```python
from build123d import *

# Parameters (mm, degrees)
SKETCH1_W                = 30
SKETCH1_H                = 30
BOSS_EXTRUDE1_DEPTH      = 30
SKETCH2_R                = 3.375
CUT_EXTRUDE1_DEPTH       = 64.639610307
FILLET1_R                = 2.5
CUT_EXTRUDE2_DEPTH       = 64.639610307
CIRPATTERN1_COUNT        = 4
CIRPATTERN1_COPY_1_DEPTH = 64.639610307
CIRPATTERN1_COPY_2_DEPTH = 64.639610307
CIRPATTERN1_COPY_3_DEPTH = 64.639610307


with BuildPart() as part:
    # Sketch1 → Boss-Extrude1 (new, symmetric)
    with BuildSketch(Plane.XY):
        Rectangle(SKETCH1_W, SKETCH1_H)
    extrude(amount=BOSS_EXTRUDE1_DEPTH, both=True)

    # Sketch2 → Cut-Extrude1 (cut, through all)
    with BuildSketch(Plane.XY.offset(30)):
        Circle(SKETCH2_R)
    extrude(amount=-CUT_EXTRUDE1_DEPTH, mode=Mode.SUBTRACT)

    # Fillet1
    fillet1_edges = [part.edges().sort_by_distance(p)[0] for p in [
        (15, -15, 0),
        (-15, -15, 0),
        (-15, 15, 0),
        (15, 15, 0),
    ]]
    fillet(fillet1_edges, radius=FILLET1_R)

    # Sketch3 → Cut-Extrude2 (cut, through all)
    with BuildSketch(Plane.XY.offset(30)):
        Polygon((0, 15), (-5.1, 15), (-5.1, 14.2), (-4.25, 14.2), (-4.25, 13.2), (-8.375, 13.2), (-8.375, 9.9), (-5.975, 7.5), (0, 7.5), align=None)
    cut_extrude2 = extrude(amount=-CUT_EXTRUDE2_DEPTH, mode=Mode.SUBTRACT)

    # Mirror1: Cut-Extrude2 across plane
    add(cut_extrude2.mirror(Plane(origin=(0, 0, 0), x_dir=(0, 0, 1), z_dir=(1, 0, 0))), mode=Mode.SUBTRACT)

    # CirPattern1: Cut-Extrude2 ×4 about axis
    cirpattern1_axis = Axis((0, 0, 0), (0, 0, 1))
    for i in range(1, CIRPATTERN1_COUNT):
        add(cut_extrude2.rotate(cirpattern1_axis, i * 360 / CIRPATTERN1_COUNT), mode=Mode.SUBTRACT)

    # CirPattern1 copy 1 sketch → CirPattern1 copy 1 (cut, through all)
    with BuildSketch(Plane(origin=(0, 0, 30), x_dir=(0, -1, 0), z_dir=(0, 0, 1))):
        Polygon((0, -15), (-5.1, -15), (-5.1, -14.2), (-4.25, -14.2), (-4.25, -13.2), (-8.375, -13.2), (-8.375, -9.9), (-5.975, -7.5), (0, -7.5), align=None)
    extrude(amount=-CIRPATTERN1_COPY_1_DEPTH, mode=Mode.SUBTRACT)

    # CirPattern1 copy 2 sketch → CirPattern1 copy 2 (cut, through all)
    with BuildSketch(Plane.XY.offset(30)):
        Polygon((0, -15), (-5.1, -15), (-5.1, -14.2), (-4.25, -14.2), (-4.25, -13.2), (-8.375, -13.2), (-8.375, -9.9), (-5.975, -7.5), (0, -7.5), align=None)
    extrude(amount=-CIRPATTERN1_COPY_2_DEPTH, mode=Mode.SUBTRACT)

    # CirPattern1 copy 3 sketch → CirPattern1 copy 3 (cut, through all)
    with BuildSketch(Plane(origin=(0, 0, 30), x_dir=(0, 1, 0), z_dir=(0, 0, 1))):
        Polygon((0, -15), (-5.1, -15), (-5.1, -14.2), (-4.25, -14.2), (-4.25, -13.2), (-8.375, -13.2), (-8.375, -9.9), (-5.975, -7.5), (0, -7.5), align=None)
    extrude(amount=-CIRPATTERN1_COPY_3_DEPTH, mode=Mode.SUBTRACT)


solid = part.part
```
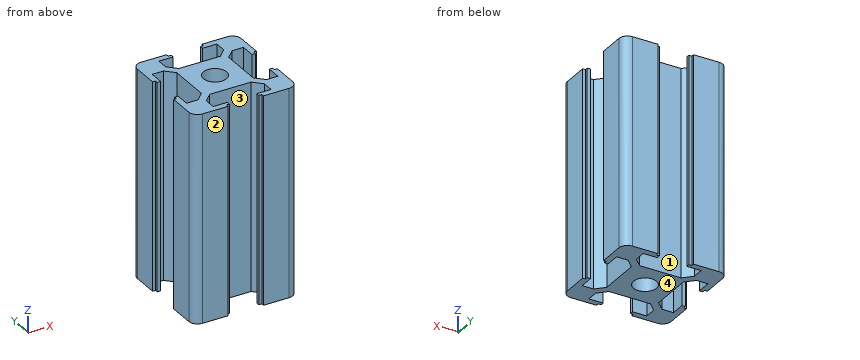
Here's how the part is built. I have some questions about the finished solid (model axes, mm). Face numbers are marked on the shaded views. A direction names the side the tool comes from. Give positions to 0.01 mm unless a question says otherwise; leave off trailing zeros. Loops run counter-clockwise (first coordinate to the right, second up) from the corner with the lowest first, then second, coordinate; pieces in that order, holes last. Notation, with made-up numbers: (41, -2) -> (100, -2) arc R30 ccw to (100, 32) -> close; hole circle Ø6 at (-21, -13.5). An arc over 180 degrees is marked (long way). Use one line per item in the form item = value. Start each with the question number.
1) Which directions (+Z, -Z, +X, -X, +Y, -Y) give clear straight access to the entire face, cutting with the end or side of a thin tool? Please do the marked faces 3 and 4.
2) Imagine slicing it at A-A (x = 0). Please give me the cut outline in (y, z) (3 decimals), then the cut area to 3 significant figures.
3) Thinking about a two-plate mould opening in X: for the marked faces 1 and 2, which applies, +X half, -X half, draft (parallel to the pull), parting line (faces both ways), or undercut?
4) Imagine slicing it at C-C (y = -6.75). Please give me the cut outline in (x, z) (3 decimals), then the cut area to 3 significant figures.
5) Please list where these lines run through material, in increasing order: line 1 along X through (y, z) = (-5, -21.5); line 2 along Y through (x, z) = (-12.5, -6) (3 decimals).
6) For P1, Ø1.1, axis at y = 13.5, z = 6.5, coming from the +X side; P2, Ø0.9, axis at x = -14.5, z = -1.5, coming from the +Y side; P3, Ø4, axis at x = -1, z = -17.5, coming from the +Y side, each with a flat end and sliding along its axis, tell me the tip position at first contact or that it passes through.
Check values:
q1.face_3 = +Z, -Z
q1.face_4 = -Z, +X, -X, +Y, -Y
q2.outline = (-7.5, -30) -> (-3.375, -30) -> (-3.375, 30) -> (-7.5, 30) -> close; (3.375, -30) -> (7.5, -30) -> (7.5, 30) -> (3.375, 30) -> close
q2.area = 495 mm^2
q3.face_1 = undercut
q3.face_2 = draft
q4.outline = (-15, -30) -> (-13.2, -30) -> (-13.2, 30) -> (-15, 30) -> close; (-8.275, -30) -> (8.275, -30) -> (8.275, 30) -> (-8.275, 30) -> close; (13.2, -30) -> (15, -30) -> (15, 30) -> (13.2, 30) -> close
q4.area = 1,210 mm^2
q5.line_1 = -14.2 to -13.2, -7.5 to 7.5, 13.2 to 14.2
q5.line_2 = -15 to -8.375, 8.375 to 15
q6.P1 = 14.96
q6.P2 = 14.46
q6.P3 = 7.5
